```python
from build123d import *

# Parameters (mm, degrees)
F0_R     = 5.8
F1_DEPTH = 1.8
F2_R     = 5.8
F2_R_2   = 4.7
F3_DEPTH = 0.4
F4_R     = 4.7
F5_DEPTH = 1.8
F6_R     = 5.8
F6_R_2   = 4.7
F6_R_3   = 2
F7_DEPTH = 0.2


# Not quite as in the source:
# - a feature names something its author has since deleted; it is built from what else it names


with BuildPart() as f1:
    # F0 (on Front) → F1 (new body)
    with BuildSketch(Plane.XZ):
        Circle(F0_R)
    extrude(amount=F1_DEPTH)

    # F2 (on face) → F3 (join)
    with BuildSketch(Plane.XZ.offset(1.8)):
        Circle(F2_R)
        Circle(F2_R_2, mode=Mode.SUBTRACT)
    extrude(amount=F3_DEPTH)

    # F4 (on face) → F5 (cut)
    with BuildSketch(Plane.XZ.offset(1.8)):
        Circle(F4_R)
    extrude(amount=-F5_DEPTH, mode=Mode.SUBTRACT)

    # F6 (on face) → F7 (join)
    with BuildSketch(Plane.XZ.offset(2.2)):
        Circle(F6_R)
        Circle(F6_R_2, mode=Mode.SUBTRACT)
        Circle(F6_R_2)
        Circle(F6_R_3, mode=Mode.SUBTRACT)
    extrude(amount=F7_DEPTH)


solid = f1.part
```
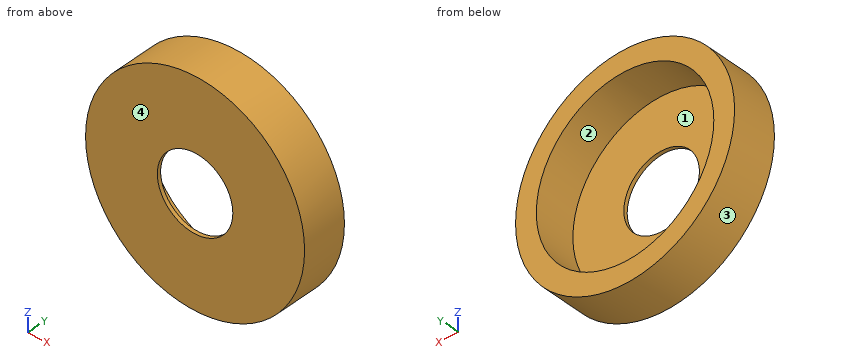
The listing builds one solid part. Answer for the finished solid, in the listing's coordinates (mm). Face numbers are marked on the shaded views. Give positions to 0.01 mm unless a question says otherwise; leave off trailing zeros. Loops run counter-clockwise (first coordinate to the right, second up) from the corner with the lowest first, then second, coordinate; pieces in that order, holes last. Notation, with made-up numbers: (87, 82) - (113, 82) arc R24 ccw to (113, 112) - close; hole circle Ø7 at (35.25, -9.75). An arc over 180 degrees is marked (long way). Return JSON: item names as keys, results as strings. Group by question number.
1. Given pin 1 Ø2.5 at (x, z) = (0, 0) entering from +Y; pin 2 Ø3 at (x, z) = (0.5, -1.5) entering from +Y, each flat-ended and moving along its own axis, determine where each tip first touches the part or whether it passes through.
2. Find section B-B (x = 0). Write down the section's boundary in (y, z), then the cut area to 3 significant figures.
3. Find section A-A (z = 0). Write down the section's boundary in (x, y).
4. Straight lines are drawn through the part: line 1 (Z direction, x = 0, y = -2.3); line 2 (Z direction, x = 0, y = -0.7); line 3 (Y direction, x = 3.25, z = -1). For each, find the intervals that lie inside material, in ascending order. Write a range as [from, to].
5. Determine the mould class of the marked faces 1, 2, 3 and 4 for opening direction Z: pulls with the +Z half, pulls with the -Z half, needs draft (parallel to the pull), parting line crosses it, or undercut.
6. Find section C-C (y = -1.15). Write down the section's boundary in (x, z), then the cut area to 3 significant figures.
7. Find section D-D (z = -4.25). Write down the section's boundary in (x, y), then the cut area to 3 significant figures.
Verdict:
{
 "1": {"pin 1": "passes through", "pin 2": "stops at y = -2.2"},
 "2": {"outline": "(-2.4, -5.8) - (0, -5.8) - (0, -4.7) - (-2.2, -4.7) - (-2.2, -2) - (-2.4, -2) - close; (-2.4, 2) - (-2.2, 2) - (-2.2, 4.7) - (0, 4.7) - (0, 5.8) - (-2.4, 5.8) - close", "area": "6.36 mm^2"},
 "3": {"outline": "(-5.8, -2.4) - (-2, -2.4) - (-2, -2.2) - (-4.7, -2.2) - (-4.7, 0) - (-5.8, 0) - close; (2, -2.4) - (5.8, -2.4) - (5.8, 0) - (4.7, 0) - (4.7, -2.2) - (2, -2.2) - close"},
 "4": {"line 1": "z = [-5.8, -2], [2, 5.8]", "line 2": "z = [-5.8, -4.7], [4.7, 5.8]", "line 3": "y = [-2.4, -2.2]"},
 "5": {"face 1": "undercut", "face 2": "undercut", "face 3": "parting line crosses it", "face 4": "needs draft"},
 "6": {"outline": "circle Ø11.6 at (0, 0); hole circle Ø9.4 at (0, 0)", "area": "36.3 mm^2"},
 "7": {"outline": "(-3.95, -2.4) - (3.95, -2.4) - (3.95, 0) - (2.01, 0) - (2.01, -2.2) - (-2.01, -2.2) - (-2.01, 0) - (-3.95, 0) - close", "area": "10.1 mm^2"}
}
